Could you check a few things on this drawing? It's one solid part, dimensions in mm from its lowest x, y, z. A direction names the side the tool comes from. Give positions to 0.01 mm unless a question says otherwise; leave off trailing zeros. Loops run counter-clockwise (first coordinate to the right, second up) from the corner with the lowest first, then second, coordinate; pieces in that order, holes last. Notation, with made-up numbers: M 5.5,55 L 12.5,55 A21 ccw 12.5,69 Z; hole C 34,86 d6. An arc over 180 degrees is marked long. Answer as a JSON object with one key per item and string values.
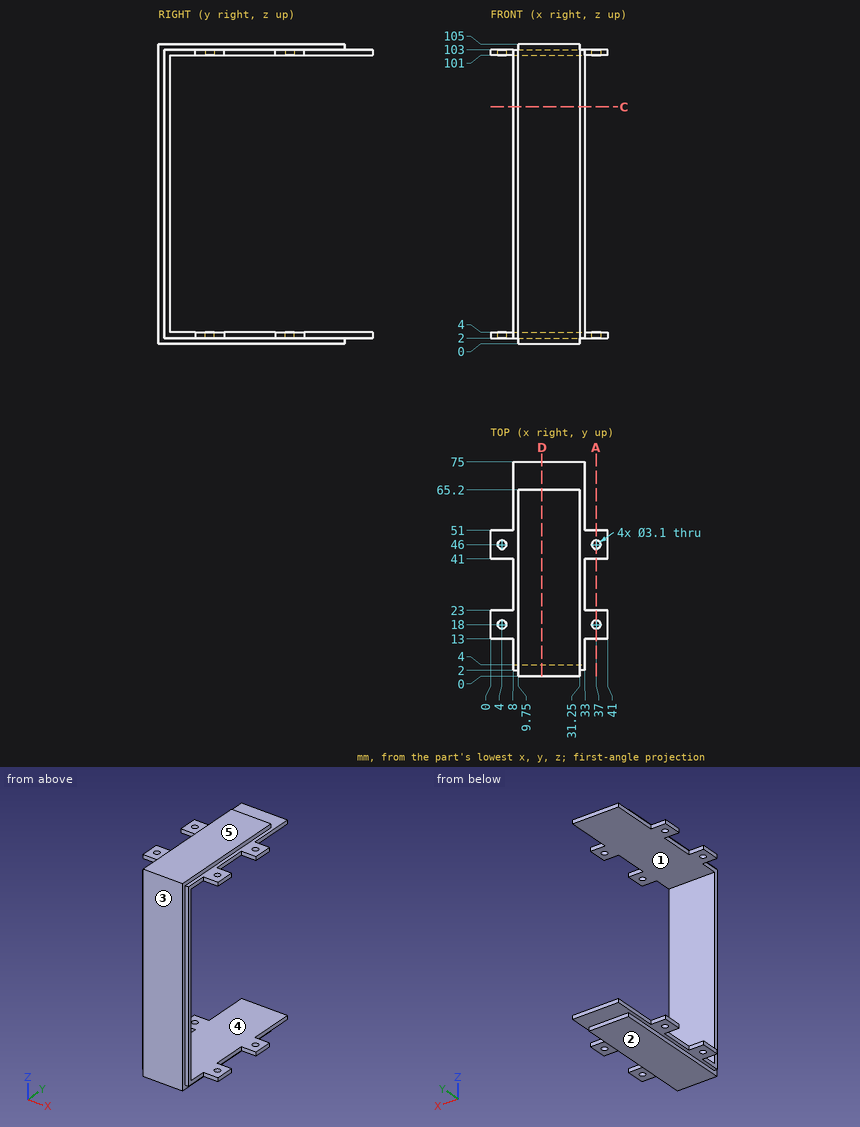
1) If we mould it in two halves opening along Z, with no side actions, what happens to the marked faces 1, 2 and 3? For each: +Z half, -Z half, draft (parallel to the pull), parting line (faces both ways), or undercut.
Answer list:
{"face 1": "undercut", "face 2": "-Z half", "face 3": "draft"}
2) Suppose I cut it at D-D, the plane x = 18. Write out the boundary of the cut face in (y, z), and give its area (3 significant figures).
Answer list:
{"outline": "M 0,0 L 65.2,0 L 65.2,2 L 75,2 L 75,4 L 4,4 L 4,101 L 75,101 L 75,103 L 65.2,103 L 65.2,105 L 0,105 Z", "area": "949 mm^2"}
3) Suppose I cut it at C-C, the plane z = 83. Write out the boundary of the cut face in (x, y), and give its area (3 significant figures).
Answer list:
{"outline": "M 8,2 L 9.75,2 L 9.75,0 L 31.25,0 L 31.25,2 L 33,2 L 33,4 L 8,4 Z", "area": "93.0 mm^2"}
4) For the marked faces 4 and 5, which set-ups out of +Z, -Z, +X, -X, +Y, -Y let a thin tool reach every point of the face, with its end or its side?
Answer list:
{"face 4": "+X, -X, +Y", "face 5": "+Z, +X, -X, +Y, -Y"}
5) Will these pins go through, and if not, where does the flat tip stop? pin 1 Ø2 at (x, y) = (32.5, 30) entering from +Z; pin 2 Ø2 at (x, z) = (5, 3.5) entering from +Y; pin 3 Ø5 at (x, y) = (4, 46) entering from -Z; pin 4 Ø1.5 at (x, y) = (35.5, 30) entering from -Z.
Answer list:
{"pin 1": "z = 103", "pin 2": "y = 51", "pin 3": "z = 2", "pin 4": "through"}
6) Please list where these lines run through material, in increasing order: line 1 along Y through (x, z) = (37, 102); line 2 along Z through (x, y) = (18.5, 40); line 3 along Z through (x, y) = (9, 65). Write a range as from..to.
Answer list:
{"line 1": "13..16.45, 19.55..23, 41..44.45, 47.55..51", "line 2": "0..4, 101..105", "line 3": "2..4, 101..103"}
7) Suppose I cut it at A-A, the plane x = 37. Give the number of separate pieces and of enclosed holes in the cut face, and give its area (3 significant figures).
Answer list:
{"separate pieces": "8", "enclosed holes": "0", "area": "55.2 mm^2"}
